For this review, take the finished solid that the model builds, in its own axes (mm). A direction names the side the tool comes from. Coordinates: 2 decimals unless noted, no trailing zeros. Loops run counter-clockwise (first coordinate to the right, second up) from the corner with the lowest first, then second, coordinate; pieces in that order, holes last. Notation, with made-up numbers: (42, 64) -> (46, 64) arc R12 ccw to (46, 87) -> close; hole circle Ø9 at (-29.75, 48.25). An arc over 180 degrees is marked (long way). Use a Markdown table: item, result.
from build123d import *

# Parameters (mm, degrees)
BOSS_EXTRUDE1_DEPTH     = 8.89
SKETCH3_R               = 6.35
BOSS_EXTRUDE2_DEPTH     = 2.54
SKETCH4_W               = 1.5875
SKETCH4_H               = 0.79375
CUT_EXTRUDE1_REACH      = 16.991
SKETCH6_R               = 2
ADVANCEDHOLE1_START     = -6.35
ADVANCEDHOLE1_OUTLINE_R = 1.25
ADVANCEDHOLE1_DEPTH     = 12.7


# Read off the part's stored shape, not the designer's step: AdvancedHole1
with BuildPart() as part:
    # Sketch2 → Boss-Extrude1 (new body)
    with BuildSketch(Plane(origin=(0, 0, 0), x_dir=(0, 0, -1), z_dir=(1, 0, 0))):
        Polygon((7.332348419, 0), (3.666174209, 6.35), (-3.666174209, 6.35), (-7.332348419, 0), (-3.666174209, -6.35), (3.666174209, -6.35), align=None)
    extrude(amount=BOSS_EXTRUDE1_DEPTH)

    # Sketch3 → Boss-Extrude2 (add)
    with BuildSketch(Plane(origin=(8.89, 0, 0), x_dir=(0, 0, -1), z_dir=(1, 0, 0))):
        with Locations(Location((0, 0, 0), (0, 0, 150))):
            Circle(SKETCH3_R)
    extrude(amount=BOSS_EXTRUDE2_DEPTH)

    # Sketch4 → Cut-Revolve1 (revolve, cut)
    with BuildSketch(Plane.XY, mode=Mode.PRIVATE) as cut_revolve1_sk:
        with Locations((9.68375, 5.953125)):
            Rectangle(SKETCH4_W, SKETCH4_H)
    revolve(cut_revolve1_sk.sketch.rotate(Axis((0, 0, 0), (1, 0, 0)), 90), axis=Axis((0, 0, 0), (1, 0, 0)), mode=Mode.SUBTRACT)

    # Sketch6 → Cut-Extrude1 (cut, up to next)
    with BuildSketch(Plane(origin=(11.43, 0, 0), x_dir=(0, 0, -1), z_dir=(1, 0, 0)), mode=Mode.PRIVATE) as cut_extrude1_sk1:
        Circle(SKETCH6_R)
    cut_extrude1_tool1 = extrude(cut_extrude1_sk1.sketch, amount=-CUT_EXTRUDE1_REACH, mode=Mode.PRIVATE) & part.part
    add(cut_extrude1_tool1.solids().sort_by_distance((11.43, 0, 0))[0], mode=Mode.SUBTRACT)

    # AdvancedHole1 outline → AdvancedHole1 (cut)
    with BuildSketch(Plane(origin=(0, 0, 0), x_dir=(1, 0, 0), z_dir=(0, 1, 0)).offset(ADVANCEDHOLE1_START)):
        with Locations((3.175, 0)):
            Circle(ADVANCEDHOLE1_OUTLINE_R)
    extrude(amount=ADVANCEDHOLE1_DEPTH, mode=Mode.SUBTRACT)


solid = part.part
(1) For faces 1 (the face through (8.89, 1.9, -5.4)), 2 (the face through (10.95, 4.68, -4.29)), 3 (the face through (4.383, -3.219, -5.474)), list the 3-axis set-ups (+Z, -Z, +X, -X, +Y, -Y) from which the entire face can be reached by the end or side of a thin tool; tool diameter is ignored.
Found:
| item | result |
|---|---|
| face 1 | none |
| face 2 | +X |
| face 3 | -Z, +X, -X, -Y |
(2) Take a section at B-B on x = 5. Write out the cut boundary in (y, z), plus the area to 3 significant figures.
Found:
| item | result |
|---|---|
| outline | (-6.35, -3.67) -> (0, -7.33) -> (6.35, -3.67) -> (6.35, 3.67) -> (0, 7.33) -> (-6.35, 3.67) -> close; hole circle Ø4 at (0, 0) |
| area | 127 mm^2 |
(3) Take a section at D-D on y = -0.75. Write out the cut boundary in (x, z).
Found:
| item | result |
|---|---|
| outline | (0, -6.9) -> (8.89, -6.9) -> (8.89, -5.51) -> (10.48, -5.51) -> (10.48, -6.31) -> (11.43, -6.31) -> (11.43, -1.85) -> (0, -1.85) -> close; (0, 1.85) -> (11.43, 1.85) -> (11.43, 6.31) -> (10.48, 6.31) -> (10.48, 5.51) -> (8.89, 5.51) -> (8.89, 6.9) -> (0, 6.9) -> close |
(4) For line 1 along Y through (x, z) = (10, 0); line 2 along X through (y, z) = (-2.25, 5.5); line 3 along X through (y, z) = (-5.25, 0) (3 decimals), list the stretches that pass through material, from the lowest coordinate up.
Found:
| item | result |
|---|---|
| line 1 | y = -5.56 to -2, 2 to 5.56 |
| line 2 | x = 0 to 8.89, 10.48 to 11.43 |
| line 3 | x = 0 to 1.925, 4.425 to 11.43 |
(5) Mouldability with a two-part tool opening along X and no side actions: class faces 4 (the face through (0, 2, -2)), 5 (the face through (4.4, -6.35, -0.8)), 6 (the face through (1.926, -3.989, -0.055)) as pulls with the +X half, pulls with the -X half, needs draft (parallel to the pull), parting line crosses it, or undercut.
Found:
| item | result |
|---|---|
| face 4 | pulls with the -X half |
| face 5 | needs draft |
| face 6 | undercut |
(6) For pin 1 Ø5 at (y, z) = (0, 0) entering from +X; pin 2 Ø2 at (x, z) = (3.175, 0) entering from -Y; pin 3 Ø1.5 at (x, y) = (9.5, -3) entering from +Z; pin 4 Ø3 at (x, y) = (6, 2.5) entering from +Z (3 decimals), all flat-tipped, find the tip position at first contact; note any pin that passes through.
Found:
| item | result |
|---|---|
| pin 1 | stops at x = 11.43 |
| pin 2 | passes through |
| pin 3 | stops at z = 5.85 |
| pin 4 | stops at z = 6.755 |
(7) Take a section at A-A on z = 0. State how many separate pieces and enclosed holes the cut face has, plus the area to 3 significant figures.
Found:
| item | result |
|---|---|
| separate pieces | 4 |
| enclosed holes | 0 |
| area | 75.2 mm^2 |
